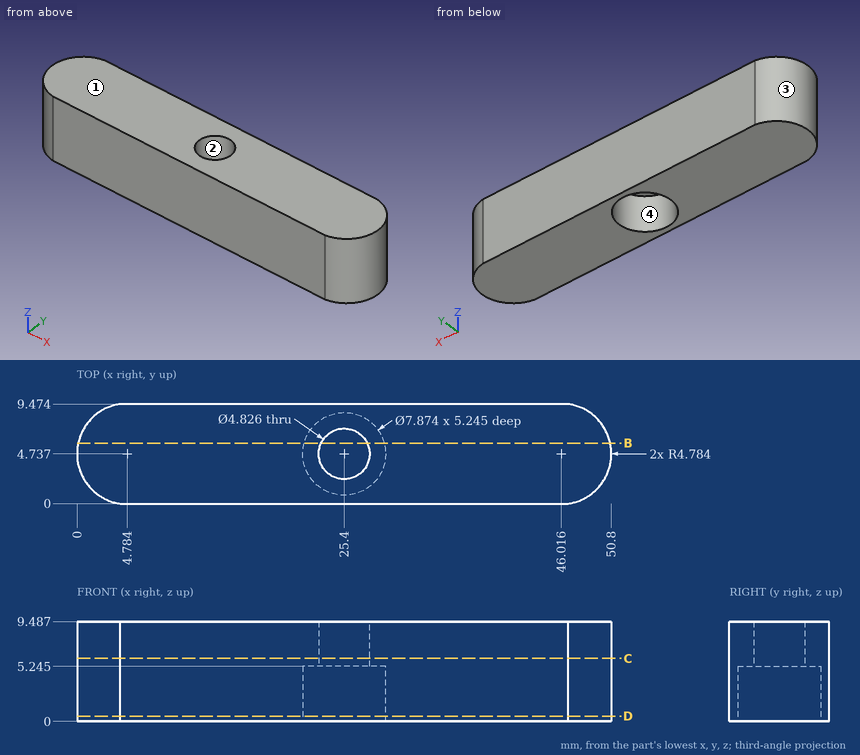
For this review, use the dimensioned drawing (mm, ordinates from the lowest corner) and the shaded views. Coordinates: 2 decimals unless noted, no trailing zeros. Loops run counter-clockwise (first coordinate to the right, second up) from the corner with the lowest first, then second, coordinate; pieces in that order, holes last. Notation, with made-up numbers: (-36, 70) - (-3, 70) arc R17 ccw to (-3, 83) - close; hole circle Ø5 at (56.5, -3.5). An arc over 180 degrees is marked (long way). Use one line per item in the form item = value. Start each with the question number.
1) Take a section at B-B (y = 5.75). State the section outline as (x, z) points (1 decimal).
2) Take a section at C-C (z = 6). State the section outline as (x, y) points, plus the area to 3 significant figures.
3) Take a section at D-D (z = 0.5). State the section outline as (x, y) points, plus the area to 3 significant figures.
4) Draft analysis for pull direction X (two halves, no side actions). For the marked faces 1, 2, 3 and 4, state which applies: released by +X, released by -X, zero draft, split by the parting line, or undercut.
5) To check wall thickness, follow probe 1 along Y at (x, z) = (25.4, 4.2); probe 2 along X at (y, z) = (4, 1.5); probe 3 along X at (y, z) = (6, 5). State the ranges of each line that lie inside material, in increasing order. Write a range as from..to.
From the geometry:
q1.outline = (0.1, 0) - (21.6, 0) - (21.6, 5.2) - (23.2, 5.2) - (23.2, 9.5) - (0.1, 9.5) - close; (27.6, 5.2) - (29.2, 5.2) - (29.2, 0) - (50.7, 0) - (50.7, 9.5) - (27.6, 9.5) - close
q2.outline = (4.12, 0) - (46.68, 0) arc R4.78 ccw to (46.68, 9.47) - (4.12, 9.47) arc R4.78 ccw to start; hole circle Ø4.83 at (25.4, 4.74)
q2.area = 444 mm2
q3.outline = (4.12, 0) - (46.68, 0) arc R4.78 ccw to (46.68, 9.47) - (4.12, 9.47) arc R4.78 ccw to start; hole circle Ø7.87 at (25.4, 4.74)
q3.area = 414 mm2
q4.face_1 = zero draft
q4.face_2 = undercut
q4.face_3 = released by -X
q4.face_4 = undercut
q5.probe_1 = 0..0.8, 8.67..9.47
q5.probe_2 = 0.06..21.53, 29.27..50.74
q5.probe_3 = 0.17..21.67, 29.13..50.63
